from build123d import *

# Parameters (mm, degrees)
BOSS_EXTRUDE1_DEPTH = 152.4
FILLET1_R           = 3.175


with BuildPart() as part:
    # Sketch3 → Boss-Extrude1 (new, symmetric)
    with BuildSketch(Plane.XY):
        Polygon((-34.925, 50.8), (3.175, 50.8), (3.175, 3.175), (13.716, 3.175), (13.716, 0), (0, 0), (0, 47.625), (-34.925, 47.625), align=None)
    extrude(amount=BOSS_EXTRUDE1_DEPTH, both=True)

    # Fillet1
    fillet1_edges = [part.edges().sort_by_distance(p)[0] for p in [
        (-34.925, 47.625, 0),
        (0, 47.625, 0),
        (0, 0, 0),
    ]]
    fillet(fillet1_edges, radius=FILLET1_R - 0.0001)  # a hair under: the kernel refuses the full size


solid = part.part
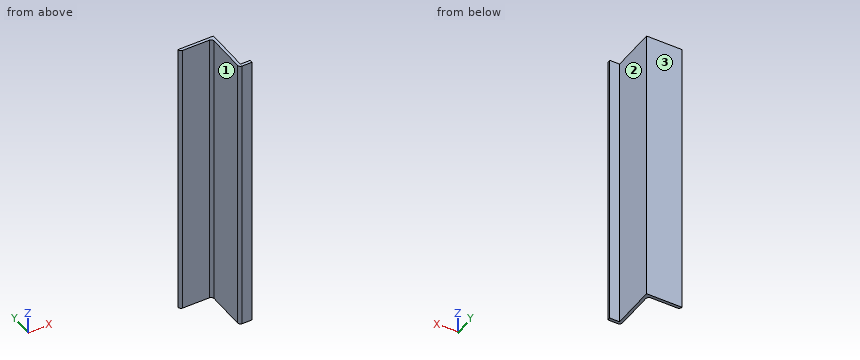
Work out the finished part from the listing and answer in its coordinate system (mm). Face numbers are marked on the shaded views. A direction names the side the tool comes from. Coordinates: 2 decimals unless noted, no trailing zeros. Loops run counter-clockwise (first coordinate to the right, second up) from the corner with the lowest first, then second, coordinate; pieces in that order, holes last. Notation, with made-up numbers: (61.25, -12) -> (79.25, -12) arc R18 cw to (79.25, -2) -> close; hole circle Ø10 at (-34.75, 24). An arc over 180 degrees is marked (long way). Write each question's results on one line, items separated by ' | '. Start each with the question number.
1) Find section B-B on x = -6. Determine the outline of the cut face in (y, z) (3 decimals).
2) Consider line 1 along X through (y, z) = (5, 103) (3 decimals); line 2 along Y through (x, z) = (-11, 99) (3 decimals); line 3 along X through (y, z) = (3, 131). Determine where each line is inside the solid, lowest interval first.
3) Flat-ended cylindrical pins translate along their axes: P1, Ø1.5, axis at y = 45.5, z = -44.5, coming from the -X side; P2, Ø12, axis at x = -24, z = 81, coming from the -Y side (3 decimals); P3, Ø2, axis at y = 17, z = -93.5, coming from the +X side (3 decimals). Find the tip coordinate at first contact, or state that the pin passes through.
4) Find section C-C on y = 23. Determine the outline of the cut face in (x, z) (3 decimals), then the cut area to 3 significant figures.
5) For the marked faces 1, 2 and 3, determine the directions among +Z, -Z, +X, -X, +Y, -Y from which every point of the face is accessible in a straight line to the end or side of a thin tool.
Response values:
1) outline: (47.625, -152.4) -> (50.8, -152.4) -> (50.8, 152.4) -> (47.625, 152.4) -> close
2) line 1: x = 0 to 3.175 | line 2: y = 47.625 to 50.8 | line 3: x = 0 to 13.72
3) P1: stops at x = -0.56 | P2: stops at y = 47.625 | P3: stops at x = 3.175
4) outline: (0, -152.4) -> (3.175, -152.4) -> (3.175, 152.4) -> (0, 152.4) -> close | area: 968 mm^2
5) face 1: +Z, -Z, -X, -Y | face 2: +Z, -Z, +X, +Y | face 3: +Z, -Z, +X, -X, +Y
